```python
from build123d import *

# Parameters (mm, degrees)
SKETCH1_R           = 14
BOSS_EXTRUDE1_DEPTH = 17
CHAMFER1_SIZE       = 5
CHAMFER3_SIZE       = 2
SKETCH3_R           = 1.65
CUT_EXTRUDE1_DEPTH  = 5
SKETCH4_R           = 1.5
BOSS_EXTRUDE2_DEPTH = 5


with BuildPart() as part:
    # Sketch1 → Boss-Extrude1 (new body)
    with BuildSketch(Plane(origin=(0, 0, 0), x_dir=(1, 0, 0), z_dir=(0, 1, 0))):
        Circle(SKETCH1_R)
    extrude(amount=BOSS_EXTRUDE1_DEPTH)

    # Chamfer1
    chamfer1_edges = [part.edges().sort_by_distance(p)[0] for p in [
        (-14, 17, 0),
    ]]
    chamfer(chamfer1_edges, length=CHAMFER1_SIZE)

    # Chamfer3
    chamfer3_edges = [part.edges().sort_by_distance(p)[0] for p in [
        (-14, 0, 0),
    ]]
    chamfer(chamfer3_edges, length=CHAMFER3_SIZE)

    # Sketch3 → Cut-Extrude1 (cut)
    with BuildSketch(Plane.XZ):
        with Locations((0, 9.5)):
            Circle(SKETCH3_R)
        with Locations((0, -9.5)):
            Circle(SKETCH3_R)
        with Locations((-8, 0)):
            Circle(SKETCH3_R)
        with Locations((8, 0)):
            Circle(SKETCH3_R)
    extrude(amount=-CUT_EXTRUDE1_DEPTH, mode=Mode.SUBTRACT)

    # Sketch4 → Boss-Extrude2 (add)
    with BuildSketch(Plane(origin=(0, 17, 0), x_dir=(1, 0, 0), z_dir=(0, 1, 0))):
        Circle(SKETCH4_R)
    extrude(amount=BOSS_EXTRUDE2_DEPTH)


solid = part.part
```
Here's how the part is built. I have some questions about the finished solid (model axes, mm). A direction names the side the tool comes from. Coordinates: 2 decimals unless noted, no trailing zeros. Loops run counter-clockwise (first coordinate to the right, second up) from the corner with the lowest first, then second, coordinate; pieces in that order, holes last. Notation, with made-up numbers: (60, -23) - (70, -23) arc R25 cw to (70, -5) - close; hole circle Ø7 at (64, 50). An arc over 180 degrees is marked (long way). Answer as CSV lines item,"result".
Q1. If we section it at C-C, the plane y = 14: Write out the boundary of the cut face in (x, z).
Response:
outline,"circle Ø24 at (0, 0)"
Q2. If we section it at A-A, the plane x = 0: Write out the boundary of the cut face in (y, z).
Response:
outline,"(0, -12) - (2, -14) - (12, -14) - (17, -9) - (17, -1.5) - (22, -1.5) - (22, 1.5) - (17, 1.5) - (17, 9) - (12, 14) - (2, 14) - (0, 12) - (0, 11.15) - (5, 11.15) - (5, 7.85) - (0, 7.85) - (0, -7.85) - (5, -7.85) - (5, -11.15) - (0, -11.15) - close"
Q3. We'd pull the mould along Z, two halves only. Please class faces 4 (the face through (8, 5, 0)), 5 (the face through (0, 5, -9)), 6 (the face through (12.932, 6.93, 5.362)), 7 (the face through (0, 0, 0)): pulls with the +Z half, pulls with the -Z half, needs draft (parallel to the pull), parting line crosses it, or undercut.
Response:
face 4,"undercut"
face 5,"undercut"
face 6,"parting line crosses it"
face 7,"needs draft"
Q4. For pin 1 (3 mm diameter, centred on x = -8, z = 0, fed in from -Y); pin 2 (3 mm diameter, centred on x = -3, y = 12.5, fed in from +Z); pin 3 (3 mm diameter, centred on x = -2, y = 17, fed in from -Z); pin 4 (1 mm diameter, centred on x = -9, y = 19, fed in from -Z), each with a flat end and sliding along its axis, tell me the tip position at first contact or that it passes through.
Response:
pin 1,"y = 5"
pin 2,"z = 13.91"
pin 3,"z = -10.33"
pin 4,"through"
Q5. For faces 1 (the face through (0, 22, 0)), 2 (the face through (6.784, 2.465, 1.115)), 3 (the face through (-1.5, 19.46, -0.07)), which set-ups out of +Z, -Z, +X, -X, +Y, -Y let a thin tool reach every point of the face, with its end or its side?
Response:
face 1,"+Z, -Z, +X, -X, +Y"
face 2,"-Y"
face 3,"+Y"
Q6. If I drill on L1, parallel to Z at x = 0, y = 2.85; L2, parallel to Z at x = 0, y = 1.6; L3, parallel to Y at x = 7.25, z = -2.5, over which ranges is the centre line in solid material (lowest first)? Write a range as [from, to].
Response:
L1,"[-14, -11.15], [-7.85, 7.85], [11.15, 14]"
L2,"[-13.6, -11.15], [-7.85, 7.85], [11.15, 13.6]"
L3,"[0, 17]"
Q7. If we section it at B-B, the plane z = 0: Write out the boundary of the cut face in (x, y).
Response:
outline,"(-14, 2) - (-12, 0) - (-9.65, 0) - (-9.65, 5) - (-6.35, 5) - (-6.35, 0) - (6.35, 0) - (6.35, 5) - (9.65, 5) - (9.65, 0) - (12, 0) - (14, 2) - (14, 12) - (9, 17) - (1.5, 17) - (1.5, 22) - (-1.5, 22) - (-1.5, 17) - (-9, 17) - (-14, 12) - close"
